Here's how the part is built. I have some questions about the finished solid (model axes, mm). Round coordinates to 2 decimals unless told otherwise and drop trailing zeros. Order: outer loops, then holes, each group sorted by start corner. A loop starts at its lowest first (then second) coordinate and runs counter-clockwise, first axis right, second up. Notation, with made-up numbers: (36.25, 65) -> (90.25, 65) arc R12 cw to (90.25, 88) -> close; hole circle Ø5 at (-36.5, 25). An arc over 180 degrees is marked (long way). Use a Markdown table: item, result. Add a question column.
(1) I want a section at B-B, the plane x = 32.5. Please give me the cut outline in (y, z) (3 decimals).
(2) I want a section at A-A, the plane z = 25. Please give me the cut outline in (x, y) (3 decimals).
(3) I'm going to push flat-ended pins straight in: P1, Ø3, axis at x = 133.5, y = -2.5, coming from the +Z side; P2, Ø3, axis at x = 3.5, y = -5, coming from the -Z side; P3, Ø3, axis at y = -6.5, z = 149.5, coming from the -X side (3 decimals); P4, Ø1.5, axis at x = 78, y = -4, coming from the +Z side (3 decimals). Where does each tip first touch, or does it pass through?
(4) If I drill on probe 1 along X at (y, z) = (-6.25, 106.5) (3 decimals); probe 2 along Z at (x, y) = (79, -4) (3 decimals), over which ranges is the centre line in solid material (lowest first)?
from build123d import *

# Parameters (mm, degrees)
F0_W     = 140.49375
F0_H     = 152.4
F1_DEPTH = 9.525
F2_W     = 9.525
F2_H     = 19.05
F2_W_2   = 19.05
F2_H_2   = 9.525
F3_DEPTH = 25.4


with BuildPart() as f1:
    # F0 (on Front) → F1 (new body)
    with BuildSketch(Plane.XZ):
        with Locations((70.246875, 76.2)):
            Rectangle(F0_W, F0_H)
    extrude(amount=F1_DEPTH)

    # F2 (on face) → F3 (cut)
    with BuildSketch(Plane.XZ.offset(9.525)):
        with Locations((4.7625, 142.875)):
            Rectangle(F2_W, F2_H)
        with Locations((4.7625, 104.775)):
            Rectangle(F2_W, F2_H)
        with Locations((4.7625, 66.675)):
            Rectangle(F2_W, F2_H)
        with Locations((4.7625, 28.575)):
            Rectangle(F2_W, F2_H)
        with Locations((32.146875, 147.6375)):
            Rectangle(F2_W_2, F2_H_2)
        with Locations((70.246875, 147.6375)):
            Rectangle(F2_W_2, F2_H_2)
        with Locations((108.346875, 147.6375)):
            Rectangle(F2_W_2, F2_H_2)
        with Locations((135.73125, 142.875)):
            Rectangle(F2_W, F2_H)
        with Locations((135.73125, 104.775)):
            Rectangle(F2_W, F2_H)
        with Locations((135.73125, 66.675)):
            Rectangle(F2_W, F2_H)
        with Locations((135.73125, 28.575)):
            Rectangle(F2_W, F2_H)
    extrude(amount=-F3_DEPTH, mode=Mode.SUBTRACT)


solid = f1.part
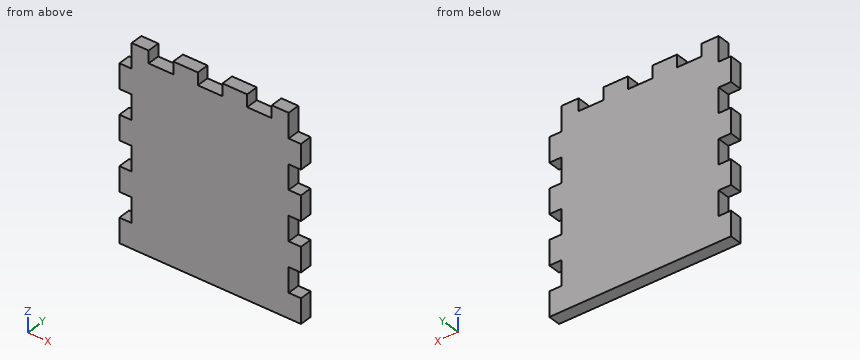
Taken from the geometry:
| question | item | result |
|---|---|---|
| 1 | outline | (-9.525, 0) -> (0, 0) -> (0, 142.875) -> (-9.525, 142.875) -> close |
| 2 | outline | (9.525, -9.525) -> (130.969, -9.525) -> (130.969, 0) -> (9.525, 0) -> close |
| 3 | P1 | stops at z = 133.35 |
| 3 | P2 | stops at z = 0 |
| 3 | P3 | stops at x = 9.525 |
| 3 | P4 | stops at z = 142.875 |
| 4 | probe 1 | x = 9.525 to 130.969 |
| 4 | probe 2 | z = 0 to 142.875 |
